Check sheet for the modelled part. Datum: model origin and axes. Units: mm. A direction names the side the tool comes from. Give positions to 0.01 mm unless a question says otherwise; leave off trailing zeros. Order: outer loops, then holes, each group sorted by start corner. A loop starts at its lowest first (then second) coordinate and runs counter-clockwise, first axis right, second up. Notation, with made-up numbers: (-34.5, 62) - (-12.5, 62) arc R26 ccw to (-12.5, 98) - close; hole circle Ø10 at (30.5, -10). An arc over 180 degrees is marked (long way). Answer in a Markdown table with one row per item.
from build123d import *

# Parameters (mm, degrees)
F0_R      = 2.75
F1_DEPTH  = 5
F5_W      = 6
F5_H      = 8.25
F7_DEPTH  = 2.751
F8_R      = 4.99999
F9_R      = 2.25
F10_DEPTH = 5.5
F11_SIZE  = 0.5


# Not quite as in the source:
# - a fillet or chamfer is up to 0.001 mm smaller than in the source, because OpenCascade refuses the exact size


with BuildPart() as f1:
    # F0 (on Front) → F1 (new body, symmetric)
    with BuildSketch(Plane.XZ):
        with BuildLine():
            ThreePointArc((-2, 41.5), (-3.5, 43), (-5, 41.5))
            Line((-5, 41.5), (-5, 29.5))
            Line((-5, 29.5), (-4, 29.5))
            Line((-4, 29.5), (-4, 22.5))
            Line((-4, 22.5), (-5, 22.5))
            Line((-5, 22.5), (-5, 0))
            ThreePointArc((-5, 0), (0, -5), (5, 0))
            Line((5, 0), (5, 13.4382623085))
            ThreePointArc((5, 13.4382623085), (5.75, 16), (5, 18.5617376915))
            Line((5, 18.5617376915), (5, 27.5))
            Line((5, 27.5), (0, 27.5))
            ThreePointArc((0, 27.5), (-1.4142135624, 28.0857864376), (-2, 29.5))
            Line((-2, 29.5), (-2, 35))
            Line((-2, 35), (-2, 37))
            Line((-2, 37), (-2, 37.25))
            Line((-2, 37.25), (-2, 39.25))
            Line((-2, 39.25), (-2, 39.5))
            Line((-2, 39.5), (-2, 41.5))
        make_face()
        Circle(F0_R, mode=Mode.SUBTRACT)
        with BuildLine():
            ThreePointArc((-2, 39.5), (-1, 40.5), (-2, 41.5))
            Line((-2, 41.5), (-2, 39.5))
        make_face()
        with BuildLine():
            ThreePointArc((-2, 37.25), (-1, 38.25), (-2, 39.25))
            Line((-2, 39.25), (-2, 37.25))
        make_face()
        with BuildLine():
            ThreePointArc((-2, 35), (-1, 36), (-2, 37))
            Line((-2, 37), (-2, 35))
        make_face()
    extrude(amount=F1_DEPTH, both=True)

    # F2 (on Front) → F3 (revolve)
    with BuildSketch(Plane.XZ):
        with BuildLine():
            Line((-3.3124492232, 25.9398471014), (-3.1381377377, 27.9322364976))
            Line((-3.1381377377, 27.9322364976), (-6.126721832, 28.1937037259))
            ThreePointArc((-6.126721832, 28.1937037259), (-7.5866085368, 27.7334032159), (-8.2934227136, 26.3756258152))
            Line((-8.2934227136, 26.3756258152), (-3.3124492232, 25.9398471014))
        make_face()
    revolve(axis=Axis((-3.9560072501, 0, 25.9961511331), (-0.9961946981, 0, 0.0871557427)))

    # F5 (on offset) → F6 (revolve, cut)
    with BuildSketch(Plane.YZ.offset(3)):
        with Locations((2, 20.125)):
            Rectangle(F5_W, F5_H)
    revolve(axis=Axis((3, 0.0511605343, 16), (0, 1, 0)), mode=Mode.SUBTRACT)

    # F5 (on offset) → F7 (cut, through all)
    with BuildSketch(Plane.YZ.offset(3)):
        with Locations((2, 20.125)):
            Rectangle(F5_W, F5_H)
    extrude(amount=F7_DEPTH, mode=Mode.SUBTRACT)

    # F8 (radius 5 in the source; OpenCascade refuses exactly that, so slightly less here)
    f8_edges = [f1.edges().sort_by_distance(p)[0] for p in [
        (5, 0, 27.5),
    ]]
    fillet(f8_edges, radius=F8_R)

    # F9 (on face) → F10 (join)
    with BuildSketch(Plane(origin=(0, -1, 0), x_dir=(-1, 0, 0), z_dir=(0, 1, 0))):
        with Locations((-3, 16)):
            Circle(F9_R)
    extrude(amount=F10_DEPTH)

    # F11
    f11_edges = [f1.edges().sort_by_distance(p)[0] for p in [
        (5.25, 4.5, 16),
    ]]
    chamfer(f11_edges, length=F11_SIZE)


solid = f1.part
(1) Gauge pin test, flat ends, axial feed: P1, Ø4.5, axis at y = 0.5, z = 31.5, coming from the +X side; P2, Ø1, axis at x = -2.5, y = 3.5, coming from the +Z side; P3, Ø2, axis at y = -3, z = 20, coming from the +X side. Record the tip position at first contact, or that the pin passes through.
Geometry says:
| item | result |
|---|---|
| P1 | x = -1.98 |
| P2 | z = 42.91 |
| P3 | x = 5 |
(2) Cross-section at C-C, the plane z = 36. Record the cut outline in (x, y), then the cut area to 3 significant figures.
Geometry says:
| item | result |
|---|---|
| outline | (-5, -5) - (-1, -5) - (-1, 5) - (-5, 5) - close |
| area | 40.0 mm² |
(3) Access from +Z, -Z, +X, -X, +Y, -Y to the whole of each face (thin tool, end or side, straight path). Record for faces 5 (the cylindrical face through (3.488, 1.465, 13.804)), 6 (the flat face through (-2, 0, 32)), 7 (the flat face through (4, 2, 24.25)).
Geometry says:
| item | result |
|---|---|
| face 5 | +Y |
| face 6 | +X, +Y, -Y |
| face 7 | +X, +Y |
(4) Cross-section at D-D, the plane z = 6. Record the cut outline in (x, y).
Geometry says:
| item | result |
|---|---|
| outline | (-5, -5) - (5, -5) - (5, 5) - (-5, 5) - close |
(5) Cross-section at B-B, the plane x = -3.5. Record the cut outline in (y, z).
Geometry says:
| item | result |
|---|---|
| outline | (-5, -3.57) - (5, -3.57) - (5, 10.92) - (-1, 10.92) - (-1, 21.08) - (5, 21.08) - (5, 43) - (-5, 43) - close |
(6) Cross-section at A-A, the plane z = 16. Record the cut outline in (x, y).
Geometry says:
| item | result |
|---|---|
| outline | (-5, -5) - (5.75, -5) - (5.75, -1) - (5.25, -1) - (5.25, 4) - (4.75, 4.5) - (1.25, 4.5) - (0.75, 4) - (0.75, -1) - (-5, -1) - close |
(7) Thickness scan on L1, parallel to Z at x = 0, y = 2; L2, parallel to Z at x = 1, y = 3.75; L3, parallel to X at y = -3.25, z = 22. Record the ranges inside material, lowest first.
Geometry says:
| item | result |
|---|---|
| L1 | -5 to -2.75, 2.75 to 8.31, 23.69 to 27.5 |
| L2 | -4.9 to -2.56, 2.56 to 8, 14.97 to 17.03, 24 to 27.4 |
| L3 | -5 to 5 |
(8) Mould release check, pull along Z, two halves, no side actions. Record for faces 1 (the cylindrical face through (0, 0, -5)), 2 (the flat face through (-1, 5, 3)), 3 (the cylindrical face through (-1, -0.1, 40.5)), 4 (the flat face through (-4, -2.3, 26)): pulls with the +Z half, pulls with the -Z half, needs draft (parallel to the pull), parting line crosses it, or undercut.
Geometry says:
| item | result |
|---|---|
| face 1 | pulls with the -Z half |
| face 2 | needs draft |
| face 3 | undercut |
| face 4 | undercut |
